```python
from build123d import *

# Parameters (mm, degrees)
SKETCH1_R           = 2.54
BOSS_EXTRUDE1_DEPTH = 3.175


with BuildPart() as part:
    # Sketch1 → Boss-Extrude1 (new body)
    with BuildSketch(Plane.XY):
        with BuildLine():
            Line((311.091686831, 197.898797126), (326.703198739, 191.301256821))
            Line((326.703198739, 191.301256821), (333.151451498, 181.876980863))
            ThreePointArc((333.151451498, 181.876980863), (337.221932682, 179.221504152), (341.977903119, 180.22206341))
            Line((341.977903119, 180.22206341), (365.723910723, 196.46949289))
            ThreePointArc((365.723910723, 196.46949289), (368.379387434, 200.539974074), (367.378828176, 205.295944512))
            Line((367.378828176, 205.295944512), (354.629507637, 223.929382055))
            ThreePointArc((354.629507637, 223.929382055), (349.230909811, 229.445982169), (342.271098909, 232.783461386))
            Line((342.271098909, 232.783461386), (324.973841412, 237.619253265))
            ThreePointArc((324.973841412, 237.619253265), (285.321700623, 308.046185122), (355.74863248, 347.698325911))
            Line((355.74863248, 347.698325911), (373.045889977, 342.862534033))
            ThreePointArc((373.045889977, 342.862534033), (401.136177569, 361.972870124), (377.568221423, 386.443682241))
            Line((377.568221423, 386.443682241), (127.710075685, 369.975787878))
            ThreePointArc((127.710075685, 369.975787878), (100.141013715, 364.248423846), (75.202698434, 351.174162585))
            Line((75.202698434, 351.174162585), (-20.489180282, 282.58567349))
            ThreePointArc((-20.489180282, 282.58567349), (-30.801832031, 237.023711212), (13.226628142, 221.411604128))
            Line((13.226628142, 221.411604128), (97.792658847, 255.734356495))
            Line((97.792658847, 255.734356495), (157.72015625, 280.057085564))
            Line((157.72015625, 280.057085564), (175.551948383, 255.17889226))
            Line((175.551948383, 255.17889226), (311.091686831, 197.898797126))
        make_face()
        with Locations((379.029877129, 364.266798159)):
            Circle(SKETCH1_R, mode=Mode.SUBTRACT)
        with Locations((336.287111757, 211.37919726)):
            Circle(SKETCH1_R, mode=Mode.SUBTRACT)
        with Locations((0, 254)):
            Circle(SKETCH1_R, mode=Mode.SUBTRACT)
    extrude(amount=BOSS_EXTRUDE1_DEPTH)


solid = part.part
```
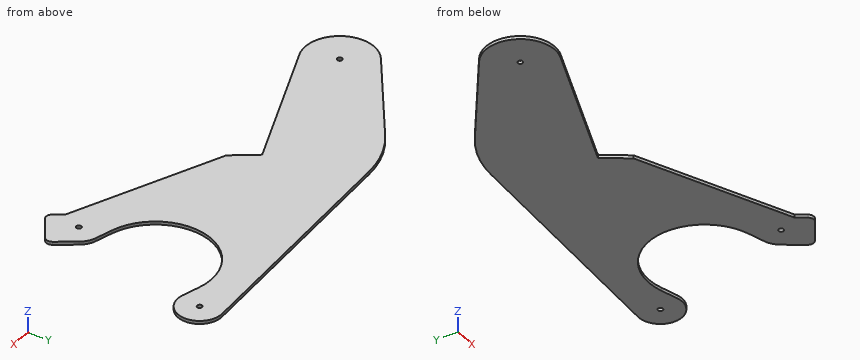
Geometry check sheet. Reference: the model listing, model coordinates, mm. Coordinates: 2 decimals unless noted, no trailing zeros. Loops run counter-clockwise (first coordinate to the right, second up) from the corner with the lowest first, then second, coordinate; pieces in that order, holes last.
Item 1: Sectioned sample at C-C, the plane x = 252. Record the boundary of the cut face in (y, z) (3 decimals).
Item 2: Thickness scan on line 1 (X direction, y = 254, z = 2); line 2 (X direction, y = 225, z = 1.95); line 3 (Y direction, x = 301, z = 2.3). Record the ranges inside material, lowest first.
Item 3: Go/stop test with flat-tipped pins: pin 1 Ø4 at (x, y) = (379.03, 364.27) entering from -Z; pin 2 Ø1.5 at (y, z) = (287.5, 2) entering from -X. Record where each tip stops, or that it passes through.
Item 4: Sectioned sample at A-A, the plane z = 1.85. Count the separate pieces of the cut face and the enclosed holes in it, then the cut area to 3 significant figures.
Item 5: Sectioned sample at B-B, the plane y = 323.5. Record the boundary of the cut face in (x, z) (3 decimals).
Check result:
1. outline: (222.871, 0) - (378.168, 0) - (378.168, 3.175) - (222.871, 3.175) - close
2. line 1: x = -35.17 to -2.54, 2.54 to 93.52, 178.34 to 298.27
2. line 2: x = -19.9 to 22.07, 246.96 to 353.85
2. line 3: y = 202.16 to 251.22, 334.09 to 381.4
3. pin 1: passes through
3. pin 2: stops at x = -14.68
4. separate pieces: 1
4. enclosed holes: 3
4. area: 43,500 mm2
5. outline: (36.593, 0) - (292.247, 0) - (292.247, 3.175) - (36.593, 3.175) - close
